Design review of the part shown in the three views and the two pictorial views. Dimensions are in mm from the part's minimum x, y and z. Coordinates: 2 decimals unless noted, no trailing zeros. Write each loop counter-clockwise with the first axis right and the second up, starting at its lowest first coordinate (ties: lowest second). Pieces come first, ordered by that corner, then holes. Notation, with made-up numbers: (49.5, 40) -> (73.5, 40) arc R25 ccw to (73.5, 67) -> close; hole circle Ø4 at (48, 31). An arc over 180 degrees is marked (long way). Write each question's results on one line, items separated by ' | '.
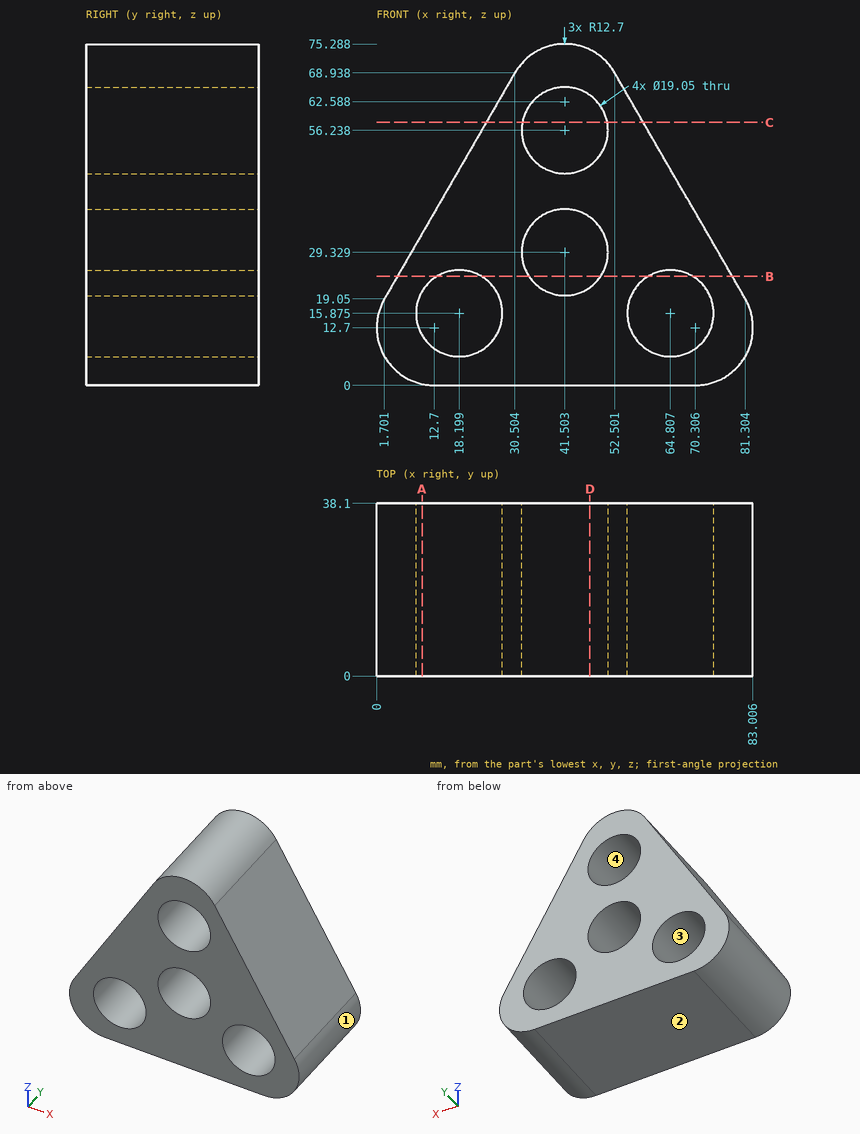
Q1. For line 1 (Z direction, x = 42, y = 32); line 2 (Z direction, x = 45, y = 31); line 3 (X direction, y = 28, z = 56) (1 decimal), list the stretches that pass through material, from the lowest coordinate up. Write a range as from..to.
Solution:
line 1: 0..19.82, 38.84..46.73, 65.75..75.28 | line 2: 0..20.47, 38.19..47.38, 65.1..74.8 | line 3: 23..32, 51..60
Q2. Add section D-D (x = 47). Write out the cut boundary in (y, z).
Solution:
outline: (0, 0) -> (38.1, 0) -> (38.1, 21.55) -> (0, 21.55) -> close; (0, 37.11) -> (38.1, 37.11) -> (38.1, 48.46) -> (0, 48.46) -> close; (0, 64.02) -> (38.1, 64.02) -> (38.1, 74.04) -> (0, 74.04) -> close
Q3. Add section A-A (x = 10). Write out the cut boundary in (y, z).
Solution:
outline: (0, 0.29) -> (38.1, 0.29) -> (38.1, 11.03) -> (0, 11.03) -> close; (0, 20.72) -> (38.1, 20.72) -> (38.1, 33.42) -> (0, 33.42) -> close
Q4. Clearance check with flat-ended pins moving along their axes: P1, Ø5, axis at y = 12.5, z = 18, coming from the +X side; P2, Ø3, axis at y = 12.5, z = 58.5, coming from the +X side (1 decimal); P3, Ø4, axis at y = 4, z = 59.5, coming from the +X side (1 decimal); P4, Ø6, axis at x = 8.5, z = 34.5, coming from the -Y side. State where each tip first meets the part, or that it passes through.
Solution:
P1: x = 82.69 | P2: x = 59.4 | P3: x = 59.1 | P4: y = 0
Q5. Draft analysis for pull direction Z (two halves, no side actions). For the marked faces 1, 2, 3 and 4, state which applies: pulls with the +Z half, pulls with the -Z half, needs draft (parallel to the pull), parting line crosses it, or undercut.
Solution:
face 1: parting line crosses it | face 2: pulls with the -Z half | face 3: undercut | face 4: undercut
Q6. Add section C-C (z = 58). Write out the cut boundary in (x, y).
Solution:
outline: (24.19, 0) -> (32.14, 0) -> (32.14, 38.1) -> (24.19, 38.1) -> close; (50.86, 0) -> (58.82, 0) -> (58.82, 38.1) -> (50.86, 38.1) -> close
Q7. Add section B-B (z = 24). Write out the cut boundary in (x, y) (1 decimal).
Solution:
outline: (4.6, 0) -> (13.2, 0) -> (13.2, 38.1) -> (4.6, 38.1) -> close; (23.2, 0) -> (33.6, 0) -> (33.6, 38.1) -> (23.2, 38.1) -> close; (49.4, 0) -> (59.8, 0) -> (59.8, 38.1) -> (49.4, 38.1) -> close; (69.8, 0) -> (78.4, 0) -> (78.4, 38.1) -> (69.8, 38.1) -> close
